Model file for the job. Use its own axes, mm. Face numbers are marked on the shaded views. A direction names the side the tool comes from. Give positions to 0.01 mm unless a question says otherwise; leave off trailing zeros. Write each loop counter-clockwise with the first axis right and the second up, starting at its lowest first coordinate (ties: lowest second). Pieces come first, ordered by that corner, then holes. Notation, with made-up numbers: M -35.75,-14.5 L -23.75,-14.5 A22 cw -23.75,22.5 Z; hole C 54,80.25 d3. An arc over 180 degrees is marked long. Answer as a JSON object with one key per item and string values. Group by question number.
```python
from build123d import *

# Parameters (mm, degrees)
SKETCH1_R           = 38.1
BOSS_EXTRUDE1_DEPTH = 12.7
SKETCH2_W           = 114.3
SKETCH2_H           = 25.4
BOSS_EXTRUDE2_DEPTH = 12.7
FILLET1_R           = 12.7
FILLET4_R           = 7.62
FILLET5_R           = 7.62


# Some blends are built 0.0001 mm under size
with BuildPart() as part:
    # Sketch1 → Boss-Extrude1 (new body)
    with BuildSketch(Plane.XY):
        Circle(SKETCH1_R)
    extrude(amount=BOSS_EXTRUDE1_DEPTH)

    # Sketch2 → Boss-Extrude2 (add)
    with BuildSketch(Plane.XY.offset(12.7)):
        with Locations((57.15, 1.312743298)):
            Rectangle(SKETCH2_W, SKETCH2_H)
    extrude(amount=BOSS_EXTRUDE2_DEPTH)

    # Fillet1
    fillet1_edges = [part.edges().sort_by_distance(p)[0] for p in [
        (0, 1.312743298, 25.4),
    ]]
    fillet(fillet1_edges, radius=FILLET1_R - 0.0001)  # a hair under: the kernel refuses the full size

    # Fillet4
    # the kernel refuses this fillet: 7.62 mm, written as the material it takes off along each edge
    with BuildSketch(Plane(origin=(114.3, -30.437256702, 12.7), x_dir=(-1, 0, 0), z_dir=(0, 1, 0))) as fillet4_piece_1:
        with BuildLine():
            CenterArc((FILLET4_R, FILLET4_R), FILLET4_R, 180, 90)
            Line((0, FILLET4_R), (0, 0))
            Line((0, 0), (FILLET4_R, 0))
        make_face()
    extrude(amount=63.5, mode=Mode.SUBTRACT)
    with BuildSketch(Plane(origin=(114.3, -30.437256702, 25.4), x_dir=(-1, 0, 0), z_dir=(0, 1, 0))) as fillet4_piece_2:
        with BuildLine():
            CenterArc((FILLET4_R, -FILLET4_R), FILLET4_R, 90, 90)
            Line((0, -FILLET4_R), (0, 0))
            Line((0, 0), (FILLET4_R, 0))
        make_face()
    extrude(amount=63.5, mode=Mode.SUBTRACT)

    # Fillet5
    fillet5_edges = [part.edges().sort_by_distance(p)[0] for p in [
        (-38.074544895, -1.392490946, 12.7),
    ]]
    fillet(fillet5_edges, radius=FILLET5_R)


solid = part.part
```
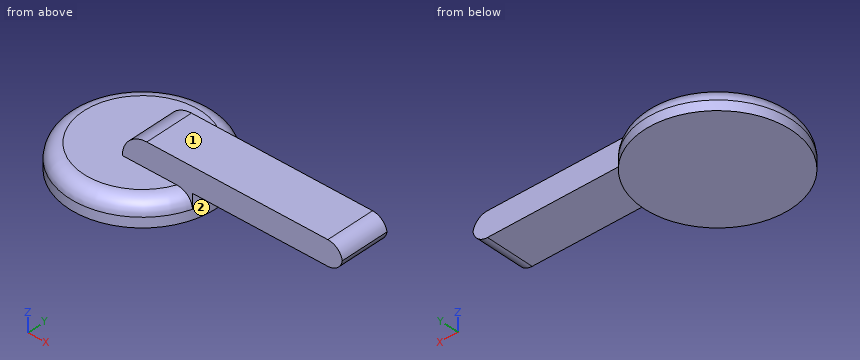
Q1. Wall check: L1, parallel to Z at x = -7, y = -10; L2, parallel to Y at x = 104, z = 20; L3, parallel to Z at x = 40, y = -10. Give the ranges that are in metal, low to high.
Q2. 3-axis set-ups, long thin cutter, end or side, ignore diameter. For the marked faces 1 and 2: which of +Z, -Z, +X, -X, +Y, -Y reach the whole face in a straight line?
Q3. Slice it at B-B, the plane z = 21.75. Write the cut outline in (x, y).
Q4. Drop flat-ended pins along their axis: P1, Ø10, axis at y = -11, z = 14.5, coming from the +X side; P2, Ø4, axis at x = 27.5, z = 13, coming from the -Y side; P3, Ø3, axis at x = -19.5, y = -8.5, coming from the +Z side; P4, Ø1.5, axis at x = 49.5, y = -8.5, coming from the -Z side. Give the stop position or say it passes through.
Solved:
{
 "1": {"L1": "z = 0 to 12.7", "L2": "y = -11.39 to 14.01", "L3": "z = 12.7 to 25.4"},
 "2": {"face 1": "+Z, +X, -X, +Y, -Y", "face 2": "-Z"},
 "3": {"outline": "M 3.79,-11.39 L 113.18,-11.39 L 113.18,14.01 L 3.79,14.01 Z"},
 "4": {"P1": "stops at x = 114.19", "P2": "stops at y = -22.75", "P3": "stops at z = 12.7", "P4": "stops at z = 12.7"}
}
